from build123d import *

# Parameters (mm, degrees)
F0_W     = 38
F0_H     = 18.5
F0_R     = 1.5
F0_W_2   = 10
F0_R_2   = 1.75
F1_DEPTH = 5
F2_W     = 25
F2_H     = 18.5
F3_DEPTH = 9.25
F5_DEPTH = 58.001


with BuildPart() as f1:
    # F0 (on Top) → F1 (new body)
    with BuildSketch(Plane.XY):
        Rectangle(F0_W, F0_H)
        with Locations((-16.65, 0)):
            Circle(F0_R, mode=Mode.SUBTRACT)
        with Locations((16.65, 0)):
            Circle(F0_R, mode=Mode.SUBTRACT)
        with Locations((24, 0)):
            Rectangle(F0_W_2, F0_H)
        with Locations((25, 0)):
            Circle(F0_R_2, mode=Mode.SUBTRACT)
        with Locations((-24, 0)):
            Rectangle(F0_W_2, F0_H)
        with Locations((-25, 0)):
            Circle(F0_R_2, mode=Mode.SUBTRACT)
    extrude(amount=F1_DEPTH)

    # F2 (on face) → F3 (join)
    with BuildSketch(Plane.XY.offset(5)):
        Rectangle(F2_W, F2_H)
    extrude(amount=F3_DEPTH)

    # F4 (on face) → F5 (cut, through all)
    with BuildSketch(Plane(origin=(-29, 0, 0), x_dir=(0, -1, 0), z_dir=(-1, 0, 0))):
        with BuildLine():
            Line((9.25, 5), (9.25, 0))
            Line((9.25, 0), (9.75, 0))
            Line((9.75, 0), (9.75, 19))
            Line((9.75, 19), (-9.25, 19))
            Line((-9.25, 19), (-9.25, 5))
            Line((-9.25, 5), (-7.7821912081, 5))
            ThreePointArc((-7.7821912081, 5), (0, 9.25), (7.7821912081, 5))
            Line((7.7821912081, 5), (9.25, 5))
        make_face()
        with BuildLine():
            ThreePointArc((7.7821912081, 5), (8.8754653026, 2.6054972006), (9.25, 0))
            Line((9.25, 0), (9.25, 5))
            Line((9.25, 5), (7.7821912081, 5))
        make_face()
        with BuildLine():
            Line((-9.25, 5), (-9.25, 0))
            ThreePointArc((-9.25, 0), (-8.8754653026, 2.6054972006), (-7.7821912081, 5))
            Line((-7.7821912081, 5), (-9.25, 5))
        make_face()
    extrude(amount=-F5_DEPTH, mode=Mode.SUBTRACT)


solid = f1.part
Input: part model. Units: mm. Frame: model coordinates. A direction names the side the tool comes from. Give positions to 0.01 mm unless a question says otherwise; leave off trailing zeros. Loops run counter-clockwise (first coordinate to the right, second up) from the corner with the lowest first, then second, coordinate; pieces in that order, holes last. Notation, with made-up numbers: M 20.25,-32.75 L 52.25,-32.75 A32 ccw 52.25,-2.75 Z; hole C 29.25,74.25 d8. An arc over 180 degrees is marked long. Use CSV: the item, a comma, the result in double quotes.
(1) Pull-direction query (Y, two-part tool) for faces 1 (the face through (23.25, 0.08, 2.46)), 2 (the face through (21, 0, 5)); classes: pulls with the +Y half, pulls with the -Y half, needs draft (parallel to the pull), parting line crosses it, or undercut.
Outcome:
face 1,"undercut"
face 2,"needs draft"
(2) Material intervals for L1, parallel to X at y = -1.25, z = 0.75; L2, parallel to Y at x = 0, z = 5; L3, parallel to X at y = -2.25, z = 7.5, sorted ascending. Write a range as [from, to].
Outcome:
L1,"x = [-29, -26.22], [-23.78, -17.48], [-15.82, 15.82], [17.48, 23.78], [26.22, 29]"
L2,"y = [-7.78, 7.78]"
L3,"x = [-12.5, 12.5]"
(3) Section B-B, the plane y = -0.75. Return loops of the section in (x, z).
Outcome:
outline,"M -29,0 L -26.58,0 L -26.58,5 L -29,5 Z; M -23.42,0 L -17.95,0 L -17.95,5 L -23.42,5 Z; M -15.35,0 L 15.35,0 L 15.35,5 L 12.5,5 L 12.5,9.22 L -12.5,9.22 L -12.5,5 L -15.35,5 Z; M 17.95,0 L 23.42,0 L 23.42,5 L 17.95,5 Z; M 26.58,0 L 29,0 L 29,5 L 26.58,5 Z"
(4) Section C-C, the plane x = 16.65. Return loops of the section in (y, z), plus the area to 3 significant figures.
Outcome:
outline,"M -9.25,0 L -1.5,0 L -1.5,5 L -7.78,5 A9.25 ccw Z; M 1.5,0 L 9.25,0 A9.25 ccw 7.78,5 L 1.5,5 Z"
area,"72.8 mm²"
(5) Section D-D, the plane z = 1.5. Return loops of the section in (x, y), plus the area to 3 significant figures.
Outcome:
outline,"M -29,-9.13 L 29,-9.13 L 29,9.13 L -29,9.13 Z; hole C -25,0 d3.5; hole C -16.65,0 d3; hole C 16.65,0 d3; hole C 25,0 d3.5"
area,"1,030 mm²"
(6) Section A-A, the plane x = 25. Return loops of the section in (y, z), plus the area to 3 significant figures.
Outcome:
outline,"M -9.25,0 L -1.75,0 L -1.75,5 L -7.78,5 A9.25 ccw Z; M 1.75,0 L 9.25,0 A9.25 ccw 7.78,5 L 1.75,5 Z"
area,"70.3 mm²"
(7) Set-up query: faces 3 (the face through (12.5, 0, 7)), 4 (the face through (-12.5, 0, 7)), 5 (the face through (29, 0, 2)). Return all of +Z, -Z, +X, -X, +Y, -Y with unobstructed straight access to the full face (end or side cutting, diameter ignored); none if empty.
Outcome:
face 3,"+Z, +X, +Y, -Y"
face 4,"+Z, -X, +Y, -Y"
face 5,"+Z, -Z, +X, +Y, -Y"
(8) Pin query (flat end, axial travel): P1, Ø3, axis at x = 14.5, z = 8, coming from the -Y side (3 decimals); P2, Ø4, axis at x = -12, y = -3, coming from the +Z side; P3, Ø8, axis at x = -21.5, y = 1, coming from the +Z side; P4, Ø1.5, axis at x = 9, z = 2, coming from the +Y side. Return the tip coordinate at first contact, or that it passes through.
Outcome:
P1,"passes through"
P2,"stops at z = 9.2"
P3,"stops at z = 5"
P4,"stops at y = 9.17"
